The drawing under review shows one solid part. Ordinate dimensions are in mm from its lowest x, y, z. Give positions to 0.01 mm unless a question says otherwise; leave off trailing zeros. Write each loop counter-clockwise with the first axis right and the second up, starting at its lowest first coordinate (ties: lowest second). Pieces come first, ordered by that corner, then holes. Notation, with made-up numbers: (2, 27.25) - (43, 27.25) arc R23 ccw to (43, 63.25) - close; hole circle Ø11 at (69, 24.5). An arc over 180 degrees is marked (long way). Write item = value, one per line.
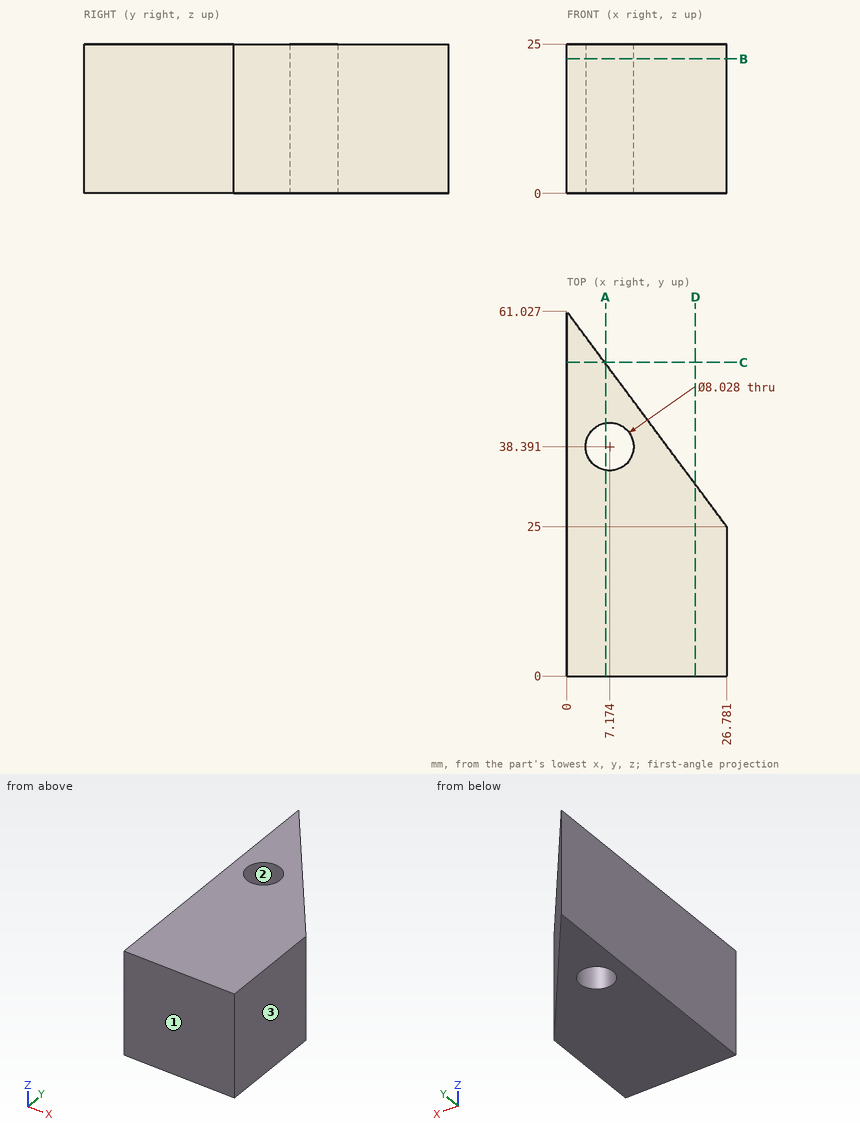
1. Take a section at D-D on x = 21.5. Give the boundary of the cut face in (y, z) (1 decimal).
Findings below:
outline = (0, 0) - (32.1, 0) - (32.1, 25) - (0, 25) - close
2. Take a section at C-C on y = 52.5. Give the boundary of the cut face in (x, z).
Findings below:
outline = (0, 0) - (6.34, 0) - (6.34, 25) - (0, 25) - close
3. Insertion check: P1, Ø1.5, axis at y = 45, z = 16, coming from the +X side; P2, Ø8, axis at x = 17, z = 20.5, coming from the +Y side; P3, Ø5, axis at x = 11.5, z = 6, coming from the +Y side. Each pin has a flat end and moves straight along its axis. Give the tip position at first contact, or say it passes through.
Findings below:
P1 = 12.47
P2 = 43.54
P3 = 48.92
4. For line 1 (Y direction, x = 7.75, z = 8.25) (1 decimal); line 2 (X direction, y = 50, z = 9); line 3 (Y direction, x = 1.5, z = 6.5), list the stretches that pass through material, from the lowest coordinate up. Write a range as from..to.
Findings below:
line_1 = 0..34.4, 42.4..50.6
line_2 = 0..8.2
line_3 = 0..59.01
5. Take a section at A-A on x = 6.5. Give the boundary of the cut face in (y, z).
Findings below:
outline = (0, 0) - (34.43, 0) - (34.43, 25) - (0, 25) - close; (42.35, 0) - (52.28, 0) - (52.28, 25) - (42.35, 25) - close
6. Draft analysis for pull direction Y (two halves, no side actions). For the marked faces 1, 2 and 3, state which applies: +Y half, -Y half, draft (parallel to the pull), parting line (faces both ways), or undercut.
Findings below:
face_1 = -Y half
face_2 = undercut
face_3 = draft
7. Take a section at B-B on z = 22.5. Give the boundary of the cut face in (x, y).
Findings below:
outline = (0, 0) - (26.78, 0) - (26.78, 25) - (0, 61.03) - close; hole circle Ø8.03 at (7.17, 38.39)
